```python
from build123d import *

# Parameters (mm, degrees)
F0_W     = 100
F0_H     = 75
F1_DEPTH = 12
F3_DEPTH = 189
F5_W     = 100
F5_H     = 75
F6_DEPTH = 12
F8_D     = 12
F8_DEPTH = 12
F8_TIP   = 3.6051637142
F9_D     = 12
F9_DEPTH = 12
F9_TIP   = 3.6051637142


with BuildPart() as f1:
    # F0 (on Top) → F1 (new body)
    with BuildSketch(Plane.XY):
        Rectangle(F0_W, F0_H)
    extrude(amount=-F1_DEPTH)

    # F2 (on face) → F3 (join)
    with BuildSketch(Plane.XY):
        with BuildLine():
            Line((-19.05, -25.4), (19.05, -25.4))
            ThreePointArc((19.05, -25.4), (23.5401280605, -23.5401280605), (25.4, -19.05))
            Line((25.4, -19.05), (25.4, 19.05))
            ThreePointArc((25.4, 19.05), (23.5401280605, 23.5401280605), (19.05, 25.4))
            Line((19.05, 25.4), (-19.05, 25.4))
            ThreePointArc((-19.05, 25.4), (-23.5401280605, 23.5401280605), (-25.4, 19.05))
            Line((-25.4, 19.05), (-25.4, -19.05))
            ThreePointArc((-25.4, -19.05), (-23.5401280605, -23.5401280605), (-19.05, -25.4))
        make_face()
        with BuildLine():
            Line((-12.7, 19.05), (12.7, 19.05))
            ThreePointArc((12.7, 19.05), (17.1901280605, 17.1901280605), (19.05, 12.7))
            Line((19.05, 12.7), (19.05, -12.7))
            ThreePointArc((19.05, -12.7), (17.1901280605, -17.1901280605), (12.7, -19.05))
            Line((12.7, -19.05), (-12.7, -19.05))
            ThreePointArc((-12.7, -19.05), (-17.1901280605, -17.1901280605), (-19.05, -12.7))
            Line((-19.05, -12.7), (-19.05, 12.7))
            ThreePointArc((-19.05, 12.7), (-17.1901280605, 17.1901280605), (-12.7, 19.05))
        make_face(mode=Mode.SUBTRACT)
    extrude(amount=F3_DEPTH)

    # F5 (on face) → F6 (join)
    with BuildSketch(Plane.XY.offset(189)):
        Rectangle(F5_W, F5_H)
        with BuildLine():
            Line((19.05, -25.4), (-19.05, -25.4))
            ThreePointArc((-19.05, -25.4), (-23.5401280605, -23.5401280605), (-25.4, -19.05))
            Line((-25.4, -19.05), (-25.4, 19.05))
            ThreePointArc((-25.4, 19.05), (-23.5401280605, 23.5401280605), (-19.05, 25.4))
            Line((-19.05, 25.4), (19.05, 25.4))
            ThreePointArc((19.05, 25.4), (23.5401280605, 23.5401280605), (25.4, 19.05))
            Line((25.4, 19.05), (25.4, -19.05))
            ThreePointArc((25.4, -19.05), (23.5401280605, -23.5401280605), (19.05, -25.4))
        make_face(mode=Mode.SUBTRACT)
        with BuildLine():
            ThreePointArc((-25.4, -19.05), (-23.5401280605, -23.5401280605), (-19.05, -25.4))
            Line((-19.05, -25.4), (19.05, -25.4))
            ThreePointArc((19.05, -25.4), (23.5401280605, -23.5401280605), (25.4, -19.05))
            Line((25.4, -19.05), (25.4, 19.05))
            ThreePointArc((25.4, 19.05), (23.5401280605, 23.5401280605), (19.05, 25.4))
            Line((19.05, 25.4), (-19.05, 25.4))
            ThreePointArc((-19.05, 25.4), (-23.5401280605, 23.5401280605), (-25.4, 19.05))
            Line((-25.4, 19.05), (-25.4, -19.05))
        make_face()
        with BuildLine():
            Line((-19.05, -12.7), (-19.05, 12.7))
            ThreePointArc((-19.05, 12.7), (-17.1901280605, 17.1901280605), (-12.7, 19.05))
            Line((-12.7, 19.05), (12.7, 19.05))
            ThreePointArc((12.7, 19.05), (17.1901280605, 17.1901280605), (19.05, 12.7))
            Line((19.05, 12.7), (19.05, -12.7))
            ThreePointArc((19.05, -12.7), (17.1901280605, -17.1901280605), (12.7, -19.05))
            Line((12.7, -19.05), (-12.7, -19.05))
            ThreePointArc((-12.7, -19.05), (-17.1901280605, -17.1901280605), (-19.05, -12.7))
        make_face(mode=Mode.SUBTRACT)
        with BuildLine():
            ThreePointArc((-12.7, 19.05), (-17.1901280605, 17.1901280605), (-19.05, 12.7))
            Line((-19.05, 12.7), (-19.05, -12.7))
            ThreePointArc((-19.05, -12.7), (-17.1901280605, -17.1901280605), (-12.7, -19.05))
            Line((-12.7, -19.05), (12.7, -19.05))
            ThreePointArc((12.7, -19.05), (17.1901280605, -17.1901280605), (19.05, -12.7))
            Line((19.05, -12.7), (19.05, 12.7))
            ThreePointArc((19.05, 12.7), (17.1901280605, 17.1901280605), (12.7, 19.05))
            Line((12.7, 19.05), (-12.7, 19.05))
        make_face()
    extrude(amount=F6_DEPTH)

    # F8
    with Locations(Plane.XY.offset(201)):
        with Locations((-38, 0), (38, 0)):
            Hole(F8_D / 2, depth=F8_DEPTH)
            with Locations((0, 0, -(F8_DEPTH + F8_TIP / 2))):  # 118° drill point
                Cone(0, F8_D / 2, F8_TIP, mode=Mode.SUBTRACT)

    # F9 (one way)
    with BuildSketch(Plane.XY):
        with Locations((-38, 22.5), (38, 22.5), (38, -22.5), (-38, -22.5)):
            Circle(F9_D / 2)
    extrude(amount=-F9_DEPTH, mode=Mode.SUBTRACT)
    with Locations(Plane.XY):
        with Locations((-38, 22.5), (38, 22.5), (38, -22.5), (-38, -22.5)):
            with Locations((0, 0, -(F9_DEPTH + F9_TIP / 2))):  # 118° drill point
                Cone(0, F9_D / 2, F9_TIP, mode=Mode.SUBTRACT)


solid = f1.part
```
Geometry check sheet. Reference: the model listing, model coordinates, mm. A direction names the side the tool comes from. Give positions to 0.01 mm unless a question says otherwise; leave off trailing zeros. Loops run counter-clockwise (first coordinate to the right, second up) from the corner with the lowest first, then second, coordinate; pieces in that order, holes last. Notation, with made-up numbers: M -24,84.25 L -4,84.25 A12 cw -4,104.25 Z; hole C -7,68 d5. An arc over 180 degrees is marked long. Write item = value, one per line. Start each with the question number.
1. Section check A-A, the plane y = 0. Enter the section's corners in (x, z).
2. Section check D-D, the plane y = 22.5. Enter the section's corners in (x, z), plus the area to 3 significant figures.
3. Section check C-C, the plane z = 123. Enter the section's corners in (x, y).
4. Go/stop test with flat-tipped pins: P1, Ø11.5, axis at x = 7, z = 123, coming from the -Y side; P2, Ø12, axis at x = 26.5, z = 172, coming from the -Y side; P3, Ø7, axis at x = -38, y = -22.5, coming from the -Z side. Record where each tip stops, or that it passes through.
5. Draft check along Y on faces 6 (the face through (-1, -37.5, -6)), 7 (the face through (0, 19.05, 93)), 8 (the face through (-50, -1, 195)). Enter one of: +Y half, -Y half, draft (parallel to the pull), parting line (faces both ways), or undercut.
6. Tool access check on faces 1 (the face through (-25.4, 0, 93)), 2 (the face through (19.05, 0, 93)), 3 (the face through (0, 25.4, 93)), 4 (the face through (-32, 0, 195)), 5 (the face through (-23.49, 23.59, 93.18)). Record the directions out of +Z, -Z, +X, -X, +Y, -Y that give a thin tool (end or side, any length) a straight path to the whole face; none if there is none.
7. Thickness scan on probe 1 along Y at (x, z) = (-38, -2); probe 2 along X at (y, z) = (0, 195); probe 3 along Z at (x, y) = (12, 33). Record the ranges inside material, lowest first.
8. Section check B-B, the plane x = -38. Enter the section's corners in (y, z).
Values follow:
q1.outline = M -50,-12 L 50,-12 L 50,0 L 25.4,0 L 25.4,189 L 32,189 L 32,201 L -32,201 L -32,189 L -25.4,189 L -25.4,0 L -50,0 Z; M -50,189 L -44,189 L -44,201 L -50,201 Z; M 44,189 L 50,189 L 50,201 L 44,201 Z; hole M -19.05,0 L 19.05,0 L 19.05,189 L -19.05,189 Z
q2.outline = M -50,-12 L -44,-12 L -44,0 L -50,0 Z; M -50,189 L -24.38,189 L -24.38,0 L -32,0 L -32,-12 L 32,-12 L 32,0 L 24.38,0 L 24.38,189 L 50,189 L 50,201 L -50,201 Z; M 44,-12 L 50,-12 L 50,0 L 44,0 Z
q2.area = 11,300 mm^2
q3.outline = M -25.4,-19.05 A6.35 ccw -19.05,-25.4 L 19.05,-25.4 A6.35 ccw 25.4,-19.05 L 25.4,19.05 A6.35 ccw 19.05,25.4 L -19.05,25.4 A6.35 ccw -25.4,19.05 Z; hole M -19.05,-12.7 A6.35 ccw -12.7,-19.05 L 12.7,-19.05 A6.35 ccw 19.05,-12.7 L 19.05,12.7 A6.35 ccw 12.7,19.05 L -12.7,19.05 A6.35 ccw -19.05,12.7 Z
q4.P1 = -25.4
q4.P2 = -25.23
q4.P3 = 189
q5.face_6 = -Y half
q5.face_7 = undercut
q5.face_8 = draft
q6.face_1 = -X, +Y, -Y
q6.face_2 = none
q6.face_3 = +X, -X, +Y
q6.face_4 = +Z
q6.face_5 = -X, +Y
q7.probe_1 = -37.5 to -28.5, -16.5 to 16.5, 28.5 to 37.5
q7.probe_2 = -50 to -44, -32 to 32, 44 to 50
q7.probe_3 = -12 to 0, 189 to 201
q8.outline = M -37.5,-12 L -28.5,-12 L -28.5,0 L -37.5,0 Z; M -37.5,189 L -6,189 L -6,201 L -37.5,201 Z; M -16.5,-12 L 16.5,-12 L 16.5,0 L -16.5,0 Z; M 6,189 L 37.5,189 L 37.5,201 L 6,201 Z; M 28.5,-12 L 37.5,-12 L 37.5,0 L 28.5,0 Z
